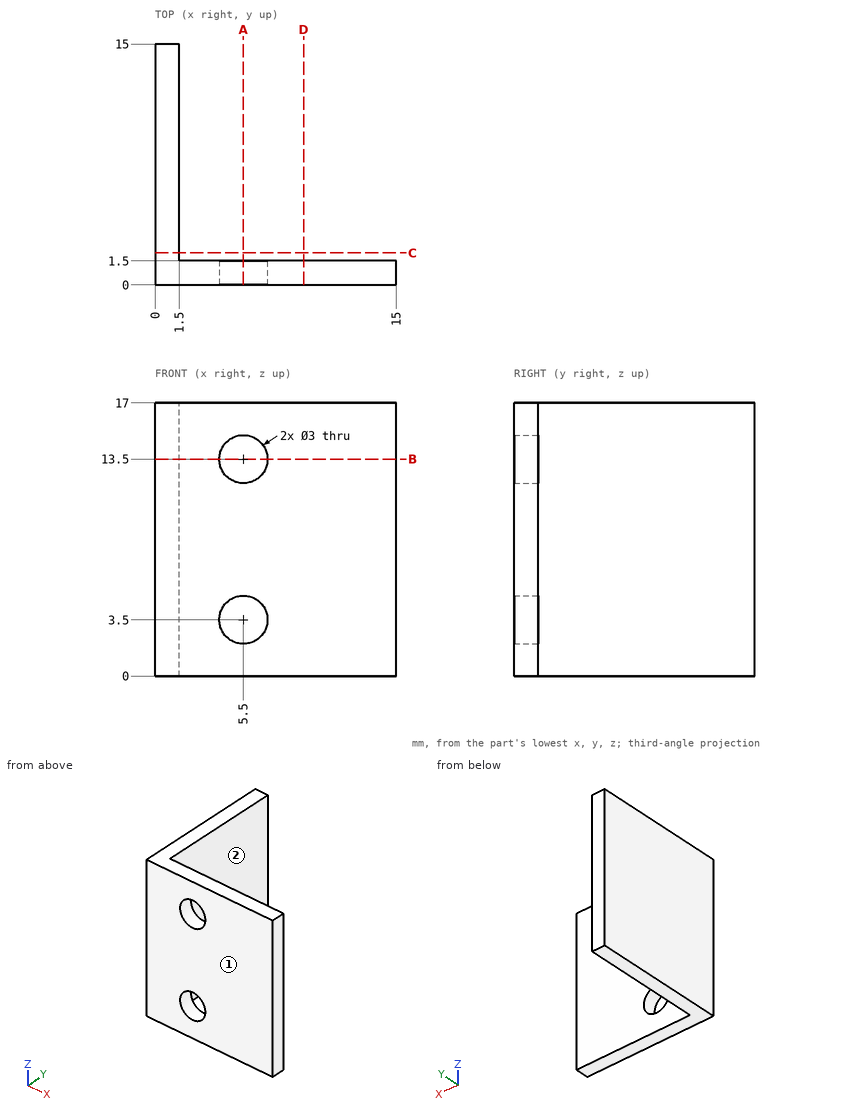
Geometry: see drawing. Coordinates: mm, zero at the bounding-box minimum. A direction names the side the tool comes from. Give positions to 0.01 mm unless a question says otherwise; leave off trailing zeros. Loops run counter-clockwise (first coordinate to the right, second up) from the corner with the lowest first, then second, coordinate; pieces in that order, holes last. Notation, with made-up numbers: M -24.5,13 L -18.5,13 A31 cw -18.5,50 Z; hole C 18,-31.75 d1. An arc over 180 degrees is marked long. Use one line per item in the form item = value.
1. Section query B-B, the plane z = 13.5. Return the cut outline in (x, y).
Numbers:
outline = M 0,0 L 4,0 L 4,1.5 L 1.5,1.5 L 1.5,15 L 0,15 Z; M 7,0 L 15,0 L 15,1.5 L 7,1.5 Z
2. First-contact query: pin 1 (8 mm diameter, centred on y = 2.5, z = 4.5, fed in from +X); pin 2 (7 mm diameter, centred on x = 9.5, z = 8, fed in from +Y); pin 3 (1.5 mm diameter, centred on y = 10, z = 6.5, fed in from +X). Flat tips, straight axial feed; report the tip coordinate or a pass-through.
Numbers:
pin_1 = 15
pin_2 = 1.5
pin_3 = 1.5
3. Reachability of the marked faces 1 and 2 from +Z, -Z, +X, -X, +Y, -Y: full face, straight path, thin tool, end or side. Return the list, or none.
Numbers:
face_1 = +Z, -Z, +X, -X, -Y
face_2 = +Z, -Z, +X, +Y
4. Section query A-A, the plane x = 5.5. Return the cut outline in (y, z), and give its area (3 significant figures).
Numbers:
outline = M 0,0 L 1.5,0 L 1.5,2 L 0,2 Z; M 0,5 L 1.5,5 L 1.5,12 L 0,12 Z; M 0,15 L 1.5,15 L 1.5,17 L 0,17 Z
area = 16.5 mm²
5. Section query C-C, the plane y = 2. Return the cut outline in (x, z).
Numbers:
outline = M 0,0 L 1.5,0 L 1.5,17 L 0,17 Z
6. Line query: L1, parallel to Z at x = 5.5, y = 0.85; L2, parallel to Y at x = 5.5, z = 7. Output: solid intervals per line, ascending.
Numbers:
L1 = 0 to 2, 5 to 12, 15 to 17
L2 = 0 to 1.5
